Autodesk Fusion 360 part; units mm, degrees
sketch "Sketch1" plane through (0, 0, 0) normal (0, 0, 1) x (1, 0, 0)
  circle A0 centre (0, 0) radius 5.25
  circle A1 centre (0, 0) radius 3.1
  circle A2 centre (0, 0) radius 1.8
  circle A3 centre (0, 0) radius 3.4
  circle A4 centre (0, 0) radius 1.5
  dimension "d1" = 10.5
  dimension "d2" = 6.2
  dimension "d3" = 3.6
  dimension "d21" = 0.3
  dimension "d22" = 0.3
extrude "Extrude1" add sketch "Sketch1" along normal blind 9.5 contours A1
extrude "Extrude2" add sketch "Sketch1" along normal blind 2 contours A0 | A3
extrude "Extrude3" add sketch "Sketch1" along normal blind 4 and the other way blind -5 contours A3
chamfer "Chamfer1" distance 0.2 angle 45 2 edges at (-3.1699, -1.2295, 4) (-3.1699, -1.2295, 5)
chamfer "Chamfer2" distance 0.5 angle 45 1 edges at (-1.6782, 0.6509, 0)
extrude "Extrude4" add sketch "Sketch1" along normal blind 5 and the other way blind -4 contours A2
chamfer "Chamfer3" distance 0.2 angle 45 2 edges at (-1.3985, 0.5424, 5) (-1.3985, 0.5424, 4)
equation "d2 = OuterRadius"
equation "d3 = InnerRadius"
equation "d21 = NotchThickness"
equation "d22 = NotchThickness"
equation "InnerRadius = 3.6 mm"
equation "OuterRadius = 6.2 mm"
equation "NotchThickness = 0.30 mm"
Read the model definition and answer for the solid it produces. Units are mm, in the model's axes. A direction names the side the tool comes from. Round coordinates to 2 decimals unless told otherwise and drop trailing zeros. Write each loop counter-clockwise with the first axis right and the second up, starting at its lowest first coordinate (ties: lowest second). Pieces come first, ordered by that corner, then holes. Notation, with made-up numbers: M 5,-26.75 L 43,-26.75 A16 cw 43,-17.75 Z; hole C 49,61 d8. An arc over 180 degrees is marked long. One line per item, written item: value.
Q1. Find section B-B on y = -4.5. Write down the section's boundary in (x, z).
Data:
outline: M -2.7,0 L 2.7,0 L 2.7,2 L -2.7,2 Z
Q2. Straight lines are drawn through the part: line 1 (Y direction, x = 0, z = 4.6); line 2 (Y direction, x = 0, z = 1.6); line 3 (Z direction, x = -4.25, y = 1.5). For each, find the intervals that lie inside material, in ascending order. Write a range as [from, to].
Data:
line 1: [-3.4, -1.5], [1.5, 3.4]
line 2: [-5.25, -1.8], [1.8, 5.25]
line 3: [0, 2]
Q3. Flat-ended cylindrical pins translate along their axes: pin 1 Ø4 at (y, z) = (3, 2) entering from -X; pin 2 Ø1.8 at (x, y) = (0, 0) entering from -Z; pin 3 Ø1 at (x, y) = (1, -0.5) entering from -Z. Find the tip coordinate at first contact, or state that the pin passes through.
Data:
pin 1: x = -5.15
pin 2: through
pin 3: z = 4.08
Q4. Find section D-D on z = 1.5. Write down the section's boundary in (x, y), plus the area to 3 significant figures.
Data:
outline: C 0,0 d10.5; hole C 0,0 d3.6
area: 76.4 mm2
Q5. Find section A-A on z = 7. Write down the section's boundary in (x, y).
Data:
outline: C 0,0 d6.2; hole C 0,0 d3.6
Q6. Which of the six approach directions +Z, -Z, +X, -X, +Y, -Y give full straight-line access (tool end or side, diameter ignored) to faces 1 (the cylindrical face through (1.717, -0.541, 2.226)), 2 (the cylindrical face through (5, -1.6, 1)), 3 (the cylindrical face through (-0.74, -3.32, 4.5))?
Data:
face 1: -Z
face 2: +Z, -Z
face 3: +Z
